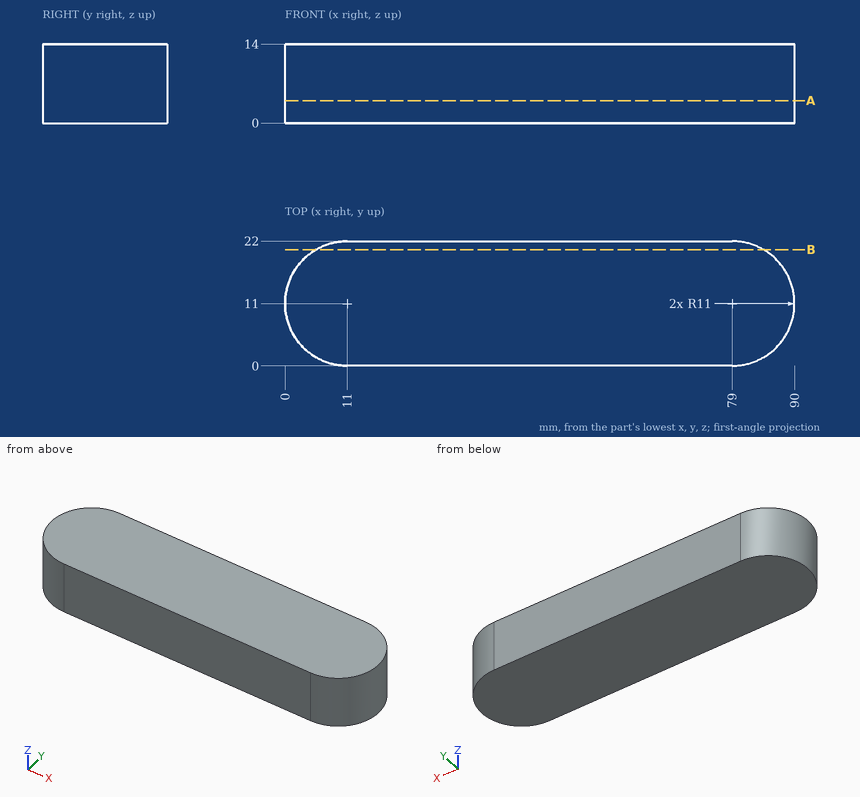
Design review of the part shown in the three views and the two pictorial views. Dimensions are in mm from the part's minimum x, y and z. Coordinates: 2 decimals unless noted, no trailing zeros. Loops run counter-clockwise (first coordinate to the right, second up) from the corner with the lowest first, then second, coordinate; pieces in that order, holes last.
Q1. For pin 1 (1.5 mm diameter, centred on y = 3.5, z = 6, fed in from +X); pin 2 (4 mm diameter, centred on y = 5.5, z = 5.5, fed in from +X), all flat-tipped, find the tip position at first contact; note any pin that passes through.
Reported:
pin 1: stops at x = 87.69
pin 2: stops at x = 89.43
Q2. To check wall thickness, follow line 1 (X direction, y = 11.5, z = 12.5); line 2 (Y direction, x = 7.5, z = 9.75); line 3 (Y direction, x = 10, z = 8.75). State the ranges of each line that lie inside material, in increasing order.
Reported:
line 1: x = 0.01 to 89.99
line 2: y = 0.57 to 21.43
line 3: y = 0.05 to 21.95
Q3. We need section B-B on y = 20.5. State the section outline as (x, z) points.
Reported:
outline: (5.45, 0) - (84.55, 0) - (84.55, 14) - (5.45, 14) - close
Q4. We need section A-A on z = 4. State the section outline as (x, y) points.
Reported:
outline: (11, 0) - (79, 0) arc R11 ccw to (79, 22) - (11, 22) arc R11 ccw to start
